from build123d import *

# Parameters (mm, degrees)
SKETCH1_W           = 25.4
SKETCH1_H           = 25.4
SKETCH1_W_2         = 22.225
SKETCH1_H_2         = 22.225
BOSS_EXTRUDE1_DEPTH = 228.6
SKETCH2_R           = 3.175
CUT_EXTRUDE1_DEPTH  = 26.4
CUT_EXTRUDE2_DEPTH  = 26.4


with BuildPart() as part:
    # Sketch1 → Boss-Extrude1 (new body)
    with BuildSketch(Plane(origin=(0, 0, 0), x_dir=(0, 0, -1), z_dir=(1, 0, 0))):
        Rectangle(SKETCH1_W, SKETCH1_H)
        Rectangle(SKETCH1_W_2, SKETCH1_H_2, mode=Mode.SUBTRACT)
    extrude(amount=BOSS_EXTRUDE1_DEPTH)

    # Sketch2 → Cut-Extrude1 (cut, through all)
    with BuildSketch(Plane.XY.offset(12.7)):
        with Locations((215.9, 0)):
            Circle(SKETCH2_R)
        with Locations((7.62, 0)):
            Circle(SKETCH2_R)
        with Locations((20.32, 0)):
            Circle(SKETCH2_R)
    extrude(amount=-CUT_EXTRUDE1_DEPTH, mode=Mode.SUBTRACT)

    # Sketch3 → Cut-Extrude2 (cut, through all)
    with BuildSketch(Plane.XY.offset(12.7)):
        with BuildLine():
            Line((228.6, 12.7), (215.9, 12.7))
            ThreePointArc((215.9, 12.7), (224.880256121, 8.980256121), (228.6, 0))
            Line((228.6, 0), (228.6, 12.7))
        make_face()
        with BuildLine():
            Line((228.6, -12.7), (228.6, 0))
            ThreePointArc((228.6, 0), (224.880256121, -8.980256121), (215.9, -12.7))
            Line((215.9, -12.7), (228.6, -12.7))
        make_face()
    extrude(amount=-CUT_EXTRUDE2_DEPTH, mode=Mode.SUBTRACT)


solid = part.part
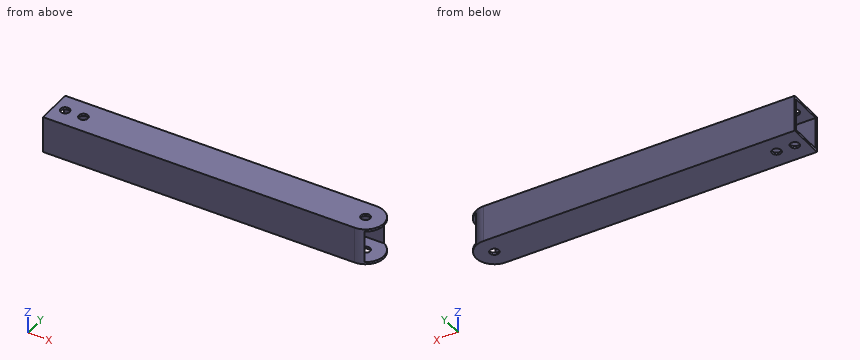
Build history of the part. All positions in model axes, mm. Coordinates: 2 decimals unless noted, no trailing zeros. Order: outer loops, then holes, each group sorted by start corner. A loop starts at its lowest first (then second) coordinate and runs counter-clockwise, first axis right, second up. Notation, with made-up numbers: (46, -31) - (86, -31) arc R34 cw to (86, 8) - close; hole circle Ø8 at (15.25, 62). An arc over 180 degrees is marked (long way). Put each result on its own line as item: value.
1. Probe line 1 along Y through (x, z) = (103.5, 9.75); line 2 along Y through (x, z) = (7.62, 12) (3 decimals). List the from-to ranges inside material, lowest first. Write a range as [from, to].
Answer sheet:
line 1: y = [-12.7, -11.11], [11.11, 12.7]
line 2: y = [-12.7, -3.175], [3.175, 12.7]
2. Saw through at D-D (x = 88.5). Write the cut outline in (y, z), and give its area (3 significant figures).
Answer sheet:
outline: (-12.7, -12.7) - (12.7, -12.7) - (12.7, 12.7) - (-12.7, 12.7) - close; hole (-11.11, -11.11) - (11.11, -11.11) - (11.11, 11.11) - (-11.11, 11.11) - close
area: 151 mm^2
3. Drop flat-ended pins along their axis: P1, Ø5.5, axis at x = 20.32, y = 0, coming from the +Z side; P2, Ø8, axis at y = 5.5, z = 9, coming from the -X side; P3, Ø10, axis at y = 9.5, z = 10, coming from the +X side. Give the stop position or say it passes through.
Answer sheet:
P1: passes through
P2: stops at x = 0
P3: stops at x = 227.73
4. Saw through at A-A (x = 7.62). Write the cut outline in (y, z) (1 decimal).
Answer sheet:
outline: (-12.7, -12.7) - (-3.2, -12.7) - (-3.2, -11.1) - (-11.1, -11.1) - (-11.1, 11.1) - (-3.2, 11.1) - (-3.2, 12.7) - (-12.7, 12.7) - close; (3.2, -12.7) - (12.7, -12.7) - (12.7, 12.7) - (3.2, 12.7) - (3.2, 11.1) - (11.1, 11.1) - (11.1, -11.1) - (3.2, -11.1) - close
5. Saw through at B-B (z = 8). Write the cut outline in (x, y), and give its area (3 significant figures).
Answer sheet:
outline: (0, -12.7) - (215.9, -12.7) arc R12.7 ccw to (222.05, -11.11) - (0, -11.11) - close; (0, 11.11) - (222.05, 11.11) arc R12.7 ccw to (215.9, 12.7) - (0, 12.7) - close
area: 699 mm^2
6. Saw through at C-C (y = 9). Write the cut outline in (x, z), and give its area (3 significant figures).
Answer sheet:
outline: (0, -12.7) - (224.86, -12.7) - (224.86, -11.11) - (0, -11.11) - close; (0, 11.11) - (224.86, 11.11) - (224.86, 12.7) - (0, 12.7) - close
area: 714 mm^2
